from build123d import *

# Parameters (mm, degrees)
BOSS_EXTRUDE1_DEPTH = 32
CHAMFER3_SIZE       = 10
CHAMFER4_SIZE       = 10
BOSS_EXTRUDE3_DEPTH = 5
SKETCH6_R           = 11
SKETCH6_R_2         = 7
BOSS_EXTRUDE4_DEPTH = 10
CUT_EXTRUDE1_START  = -10
SKETCH7_R           = 7
CUT_EXTRUDE1_DEPTH  = 10


with BuildPart() as part:
    # Sketch2 → Boss-Extrude1 (new body)
    with BuildSketch(Plane.XY):
        Polygon((4.788542225, -32.938228069), (-3.211457775, -32.938228069), (-3.211457775, 1.061771931), (-26.211457775, 1.061771931), (-26.211457775, 9.061771931), (27.788542225, 9.061771931), (27.788542225, 1.061771931), (4.788542225, 1.061771931), align=None)
    extrude(amount=BOSS_EXTRUDE1_DEPTH)

    # Chamfer3
    chamfer3_edges = [part.edges().sort_by_distance(p)[0] for p in [
        (27.788542225, 5.061771931, 32),
    ]]
    chamfer(chamfer3_edges, length=CHAMFER3_SIZE)

    # Chamfer4
    chamfer4_edges = [part.edges().sort_by_distance(p)[0] for p in [
        (-26.211457775, 5.061771931, 32),
    ]]
    chamfer(chamfer4_edges, length=CHAMFER4_SIZE)

    # Sketch5 → Boss-Extrude3 (add)
    with BuildSketch(Plane.XY):
        Polygon((27.788542225, 9.061771931), (17.788542225, 47.061771931), (-16.211457775, 47.061771931), (-26.211457775, 9.061771931), align=None)
    extrude(amount=BOSS_EXTRUDE3_DEPTH)

    # Sketch6 → Boss-Extrude4 (add)
    with BuildSketch(Plane.XY.offset(5)):
        with Locations((0, 28.061771931)):
            Circle(SKETCH6_R)
        with Locations((0, 28.061771931)):
            Circle(SKETCH6_R_2, mode=Mode.SUBTRACT)
    extrude(amount=BOSS_EXTRUDE4_DEPTH)

    # Sketch7 → Cut-Extrude1 (cut)
    with BuildSketch(Plane.XY.offset(5).offset(CUT_EXTRUDE1_START)):
        with Locations(Location((0, 28.061771931, 0), (0, 0, 180))):
            Circle(SKETCH7_R)
    extrude(amount=CUT_EXTRUDE1_DEPTH, mode=Mode.SUBTRACT)


solid = part.part
Verification items for the finished model (mm, model axes). A direction names the side the tool comes from. Coordinates: 2 decimals unless noted, no trailing zeros. Loops run counter-clockwise (first coordinate to the right, second up) from the corner with the lowest first, then second, coordinate; pieces in that order, holes last. Notation, with made-up numbers: (36.25, 70.25) -> (68.25, 70.25) arc R14 ccw to (68.25, 86.25) -> close; hole circle Ø9 at (62.25, -25). An arc over 180 degrees is marked (long way). Answer as a JSON object with one key per item and string values. Group by question number.
Item 1: Sectioned sample at D-D on z = 9. Record the boundary of the cut face in (x, y), plus the area to 3 significant figures.
Item 2: Sectioned sample at C-C on y = 27. Record the boundary of the cut face in (x, z).
Item 3: Sectioned sample at A-A on x = 0. Record the boundary of the cut face in (y, z), plus the area to 3 significant figures.
Item 4: Sectioned sample at B-B on z = 19. Record the boundary of the cut face in (x, y).
Item 5: Tool access check on faces 1 (the flat face through (7.2, 28.2, 15)), 2 (the flat face through (-3.211, -16, 16)), 3 (the flat face through (22.72, 5.12, 27.07)), 4 (the flat face through (16, 1.062, 16)). Record the directions out of +Z, -Z, +X, -X, +Y, -Y that give a thin tool (end or side, any length) a straight path to the whole face; none if there is none.
Item 6: Mould release check, pull along Y, two halves, no side actions. Record for faces 5 (the flat face through (-21.28, 5.01, 26.93)), 6 (the flat face through (-21.14, 28.33, 2.46)), 7 (the cylindrical face through (-2.385, 17.323, 9.93)): +Y half, -Y half, draft (parallel to the pull), parting line (faces both ways), or undercut.
Item 7: Scan lines: probe 1 along Y at (x, z) = (0, 11); probe 2 along Y at (x, z) = (-3.5, 13); probe 3 along Y at (x, z) = (0, 1.7). Record each from-to range of solid material in increasing order.
Item 8: Depth check by flat-ended pin: pin 1 (8 mm diameter, centred on x = -4, z = 22, fed in from -Y); pin 2 (6 mm diameter, centred on y = -6.5, z = 4.5, fed in from -X); pin 3 (11.5 mm diameter, centred on x = -14, z = 14.5, fed in from -Y); pin 4 (19 mm diameter, centred on x = 7.5, y = 25.5, fed in from +Z). Enter the tip coordinate at first touch or a pass-through.
Evaluation:
{
 "1": {"outline": "(-26.21, 1.06) -> (-3.21, 1.06) -> (-3.21, -32.94) -> (4.79, -32.94) -> (4.79, 1.06) -> (27.79, 1.06) -> (27.79, 9.06) -> (-26.21, 9.06) -> close; circle Ø22 at (0, 28.06); hole circle Ø14 at (0, 28.06)", "area": "930 mm²"},
 "2": {"outline": "(-21.49, 0) -> (-6.92, 0) -> (-6.92, 15) -> (-10.95, 15) -> (-10.95, 5) -> (-21.49, 5) -> close; (6.92, 0) -> (23.07, 0) -> (23.07, 5) -> (10.95, 5) -> (10.95, 15) -> (6.92, 15) -> close"},
 "3": {"outline": "(-32.94, 0) -> (21.06, 0) -> (21.06, 15) -> (17.06, 15) -> (17.06, 5) -> (9.06, 5) -> (9.06, 32) -> (-32.94, 32) -> close; (35.06, 0) -> (47.06, 0) -> (47.06, 5) -> (39.06, 5) -> (39.06, 15) -> (35.06, 15) -> close", "area": "1,540 mm²"},
 "4": {"outline": "(-26.21, 1.06) -> (-3.21, 1.06) -> (-3.21, -32.94) -> (4.79, -32.94) -> (4.79, 1.06) -> (27.79, 1.06) -> (27.79, 9.06) -> (-26.21, 9.06) -> close"},
 "5": {"face 1": "+Z, +X, -X, +Y", "face 2": "+Z, -Z, -X, -Y", "face 3": "+Z, +X, +Y, -Y", "face 4": "+Z, -Z, +X, -Y"},
 "6": {"face 5": "draft", "face 6": "+Y half", "face 7": "undercut"},
 "7": {"probe 1": "y = -32.94 to 9.06, 17.06 to 21.06, 35.06 to 39.06", "probe 2": "y = 1.06 to 9.06, 17.63 to 22, 34.12 to 38.49", "probe 3": "y = -32.94 to 21.06, 35.06 to 47.06"},
 "8": {"pin 1": "stops at y = -32.94", "pin 2": "stops at x = -3.21", "pin 3": "stops at y = 1.06", "pin 4": "stops at z = 15"}
}
